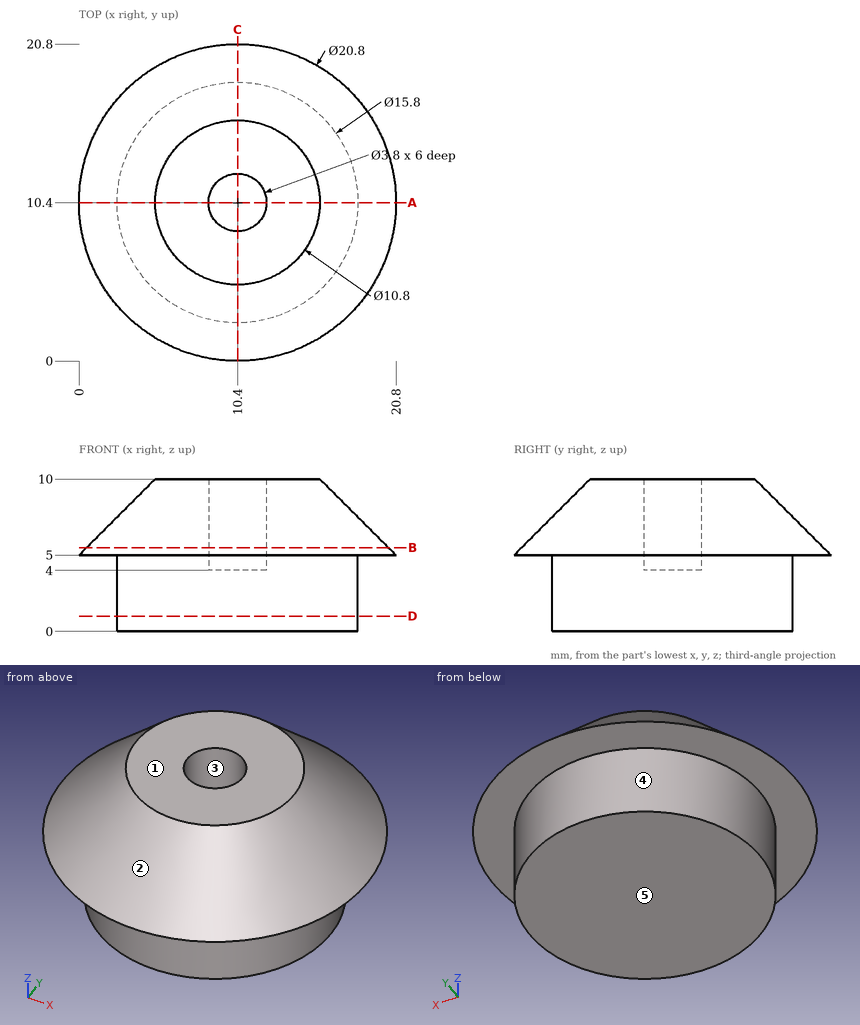
Geometry: see drawing. Coordinates: mm, zero at the bounding-box minimum. A direction names the side the tool comes from. Give positions to 0.01 mm unless a question says otherwise; leave off trailing zeros. Loops run counter-clockwise (first coordinate to the right, second up) from the corner with the lowest first, then second, coordinate; pieces in that order, holes last. Notation, with made-up numbers: (-25, 20) - (-11, 20) arc R16 cw to (-11, 27) - close; hole circle Ø1 at (67, -21). An arc over 180 degrees is marked (long way). Answer as CSV lines item,"result". Start each with the question number.
1. Pin query (flat end, axial travel): P1, Ø1, axis at y = 13.5, z = 3.5, coming from the +X side; P2, Ø1.5, axis at x = 15, z = 6, coming from the +Y side (3 decimals); P3, Ø3, axis at x = 10.5, y = 10.5, coming from the +Z side. Return the tip coordinate at first contact, or that it passes through.
2. Section A-A, the plane y = 10.4. Return loops of the section in (x, z), plus the area to 3 significant figures.
3. Section B-B, the plane z = 5.5. Return loops of the section in (x, y).
4. Reachability of the marked faces 4 and 5 from +Z, -Z, +X, -X, +Y, -Y: full face, straight path, thin tool, end or side. Return the list, or none.
5. Draft query along X for the marked faces 1, 2 and 3. Return one class per face: released by +X, released by -X, zero draft, split by the parting line, or undercut.
6. Section D-D, the plane z = 1. Return loops of the section in (x, y), plus the area to 3 significant figures.
7. Ray query, L1, parallel to X at y = 10.4, z = 8.5; L2, parallel to X at y = 10.4, z = 6.4; L3, parallel to Y at x = 16, z = 5.25. Return the intervals inside material, ascending.
Answers:
1,P1,"stops at x = 17.86"
1,P2,"stops at y = 19.525"
1,P3,"stops at z = 4"
2,outline,"(0, 5) - (2.5, 5) - (2.5, 0) - (18.3, 0) - (18.3, 5) - (20.8, 5) - (15.8, 10) - (12.3, 10) - (12.3, 4) - (8.5, 4) - (8.5, 10) - (5, 10) - close"
2,area,"135 mm2"
3,outline,"circle Ø19.8 at (10.4, 10.4); hole circle Ø3.8 at (10.4, 10.4)"
4,face 4,"-Z"
4,face 5,"-Z, +X, -X, +Y, -Y"
5,face 1,"zero draft"
5,face 2,"split by the parting line"
5,face 3,"undercut"
6,outline,"circle Ø15.8 at (10.4, 10.4)"
6,area,"196 mm2"
7,L1,"x = 3.5 to 8.5, 12.3 to 17.3"
7,L2,"x = 1.4 to 8.5, 12.3 to 19.4"
7,L3,"y = 1.93 to 18.87"
